Input: part model. Units: mm. Frame: model coordinates. A direction names the side the tool comes from. Give positions to 0.01 mm unless a question says otherwise; leave off trailing zeros. Loops run counter-clockwise (first coordinate to the right, second up) from the corner with the lowest first, then second, coordinate; pieces in that order, holes last. Notation, with made-up numbers: (-18.5, -30) - (24.5, -30) arc R26 cw to (24.5, -15) - close; hole circle Ø11 at (22.25, -1). An arc over 180 degrees is marked (long way). One line per question, with ' | ' between items. Start each with the question number.
from build123d import *

# Parameters (mm, degrees)
SCHIZZO1_W                        = 27
SCHIZZO1_H                        = 36
ESTRUSIONE_ESTRUSIONE1_DEPTH      = 4
SCHIZZO10_R                       = 1.75
TAGLIO_ESTRUSIONE5_DEPTH          = 10
SCHIZZO12_W                       = 104
SCHIZZO12_H                       = 2.549259356
ESTRUSIONE_ESTRUSIONE2_DEPTH      = 55
ESTRUSIONE_ESTRUSIONE2_DEPTH_BACK = 55
SCHIZZO14_W                       = 3
SCHIZZO14_H                       = 1.5
ESTRUSIONE_ESTRUSIONE3_DEPTH      = 110
SCHIZZO15_W                       = 27
SCHIZZO15_H                       = 4
TAGLIO_ESTRUSIONE6_DEPTH          = 5
SCHIZZO16_R                       = 13.5
TAGLIO_ESTRUSIONE7_DEPTH          = 10


with BuildPart() as part:
    # Schizzo1 → Estrusione-Estrusione1 (new body)
    with BuildSketch(Plane.XY):
        with Locations((13.5, -18)):
            Rectangle(SCHIZZO1_W, SCHIZZO1_H)
    extrude(amount=ESTRUSIONE_ESTRUSIONE1_DEPTH)

    # Schizzo10 → Taglio-Estrusione5 (cut)
    with BuildSketch(Plane.XY.offset(4)):
        with Locations((3.5, -12.5)):
            Circle(SCHIZZO10_R)
        with Locations((23.5, -12.5)):
            Circle(SCHIZZO10_R)
        with Locations((23.5, -27.5)):
            Circle(SCHIZZO10_R)
        with Locations((3.5, -27.5)):
            Circle(SCHIZZO10_R)
    extrude(amount=-TAGLIO_ESTRUSIONE5_DEPTH, mode=Mode.SUBTRACT)

    # Schizzo12 → Estrusione-Estrusione2 (add, two sides)
    with BuildSketch(Plane(origin=(13.5, 0, 0), x_dir=(0, 0, -1), z_dir=(1, 0, 0))) as estrusione_estrusione2_sk:
        with Locations((-56, -34.725370322)):
            Rectangle(SCHIZZO12_W, SCHIZZO12_H)
    extrude(amount=ESTRUSIONE_ESTRUSIONE2_DEPTH)
    extrude(estrusione_estrusione2_sk.sketch, amount=-ESTRUSIONE_ESTRUSIONE2_DEPTH_BACK)

    # Schizzo14 → Estrusione-Estrusione3 (add)
    with BuildSketch(Plane.ZY.offset(41.5)):
        with Locations((84, -32.700740644)):
            Rectangle(SCHIZZO14_W, SCHIZZO14_H)
        with Locations((99, -32.700740644)):
            Rectangle(SCHIZZO14_W, SCHIZZO14_H)
    extrude(amount=-ESTRUSIONE_ESTRUSIONE3_DEPTH)

    # Schizzo15 → Taglio-Estrusione6 (cut, through all)
    with BuildSketch(Plane.XY.offset(4)):
        with Locations((13.5, -2)):
            Rectangle(SCHIZZO15_W, SCHIZZO15_H)
    extrude(amount=-TAGLIO_ESTRUSIONE6_DEPTH, mode=Mode.SUBTRACT)

    # Schizzo16 → Taglio-Estrusione7 (cut)
    with BuildSketch(Plane(origin=(0, -33.450740644, 0), x_dir=(1, 0, 0), z_dir=(0, 1, 0))):
        with Locations((29.5, -45)):
            Circle(SCHIZZO16_R)
    extrude(amount=-TAGLIO_ESTRUSIONE7_DEPTH, mode=Mode.SUBTRACT)


solid = part.part
Q1. Section D-D, the plane x = 29.5. Output: boundary loops of the cut face in (y, z).
Q2. Section C-C, the plane z = 45. Output: boundary loops of the cut face in (x, y).
Q3. First-contact query: pin 1 (0.8 mm diameter, centred on x = -25, y = -35.5, fed in from -Z); pin 2 (1.2 mm diameter, centred on y = -21.5, z = 1.5, fed in from -X); pin 3 (1.5 mm diameter, centred on x = -9, z = 84, fed in from +Y); pin 4 (5 mm diameter, centred on x = 28, y = -21, fed in from -Z). Flat tips, straight axial feed; report the tip coordinate or a pass-through.
Q4. Section A-A, the plane x = 3.5. Output: boundary loops of the cut face in (y, z), plus the area to 3 significant figures.
Q5. Line query: L1, parallel to Y at x = 3.5, z = 2.5; L2, parallel to Z at x = 43, y = -33; L3, parallel to Z at x = 29.5, y = -35.2. Output: solid intervals per line, ascending. Write a range as from..to.
Q6. Section B-B, the plane y = -27.5. Output: boundary loops of the cut face in (x, z), plus the area to 3 significant figures.
Q7. Access query for faces 5 (the face through (-20, -35, 4)), 6 (the face through (42.377, -34.708, 40.945)), 7 (the face through (13, -31.951, 84)), 8 (the face through (14, -33.451, 44)), 9 (the face through (47, -35, 4)). Directions: +Z, -Z, +X, -X, +Y, -Y. A direction counts if a zero-diameter tool reaches every point of the face in a straight line with its end or side. Return the directions, or none.
Q8. Draft query along Y for faces 1 (the face through (13, -31.951, 99)), 2 (the face through (21.75, -12.42, 2.03)), 3 (the face through (22.21, -26.32, 2.03)), 4 (the face through (27, -20, 2)). Return one class per face: +Y half, -Y half, draft (parallel to the pull), parting line (faces both ways), or undercut.
Solved:
1) outline: (-36, 4) - (-33.45, 4) - (-33.45, 31.5) - (-36, 31.5) - close; (-36, 58.5) - (-33.45, 58.5) - (-33.45, 82.5) - (-31.95, 82.5) - (-31.95, 85.5) - (-33.45, 85.5) - (-33.45, 97.5) - (-31.95, 97.5) - (-31.95, 100.5) - (-33.45, 100.5) - (-33.45, 108) - (-36, 108) - close
2) outline: (-41.5, -36) - (16, -36) - (16, -33.45) - (-41.5, -33.45) - close; (43, -36) - (68.5, -36) - (68.5, -33.45) - (43, -33.45) - close
3) pin 1: stops at z = 4 | pin 2: stops at x = 0 | pin 3: stops at y = -31.95 | pin 4: stops at z = 0
4) outline: (-36, 0) - (-29.25, 0) - (-29.25, 4) - (-33.45, 4) - (-33.45, 82.5) - (-31.95, 82.5) - (-31.95, 85.5) - (-33.45, 85.5) - (-33.45, 97.5) - (-31.95, 97.5) - (-31.95, 100.5) - (-33.45, 100.5) - (-33.45, 108) - (-36, 108) - close; (-25.75, 0) - (-14.25, 0) - (-14.25, 4) - (-25.75, 4) - close; (-10.75, 0) - (-4, 0) - (-4, 4) - (-10.75, 4) - close | area: 374 mm²
5) L1: y = -36..-29.25, -25.75..-14.25, -10.75..-4 | L2: z = 82.5..85.5, 97.5..100.5 | L3: z = 4..31.5, 58.5..108
6) outline: (0, 0) - (1.75, 0) - (1.75, 4) - (0, 4) - close; (5.25, 0) - (21.75, 0) - (21.75, 4) - (5.25, 4) - close; (25.25, 0) - (27, 0) - (27, 4) - (25.25, 4) - close | area: 80.0 mm²
7) face 5: -Z, -X, +Y, -Y | face 6: +Y, -Y | face 7: +Z, +X, -X, +Y | face 8: +X, -X, +Y | face 9: -Z, +X, +Y, -Y
8) face 1: +Y half | face 2: undercut | face 3: undercut | face 4: draft
